from build123d import *

# Parameters (mm, degrees)
SKETCH2_W                   = 100
SKETCH2_H                   = 47
BOSS_EXTRUDE1_DEPTH         = 40
FILLET1_R                   = 10
CUT_EXTRUDE1_REACH          = 70.207
M6_TAPPED_HOLE1_D           = 5
M6_TAPPED_HOLE1_DEPTH       = 17
M6_TAPPED_HOLE1_CSINK_D     = 6.05
M6_TAPPED_HOLE1_CSINK_ANGLE = 90
M6_TAPPED_HOLE1_TIP         = 1.502151548


with BuildPart() as part:
    # Sketch2 → Boss-Extrude1 (new body)
    with BuildSketch(Plane(origin=(0, 0, 0), x_dir=(1, 0, 0), z_dir=(0, 1, 0))):
        Rectangle(SKETCH2_W, SKETCH2_H)
    extrude(amount=-BOSS_EXTRUDE1_DEPTH)

    # Fillet1
    fillet1_edges = [part.edges().sort_by_distance(p)[0] for p in [
        (50, -20, 23.5),
        (-50, -20, 23.5),
        (-50, -20, -23.5),
        (50, -20, -23.5),
    ]]
    fillet(fillet1_edges, radius=FILLET1_R)

    # Sketch3 → Cut-Extrude1 (cut, up to next)
    with BuildSketch(Plane(origin=(0, 0, 0), x_dir=(1, 0, 0), z_dir=(0, 1, 0)), mode=Mode.PRIVATE) as cut_extrude1_sk1:
        with BuildLine():
            Line((24.05, -10.14), (24.05, 10.14))
            ThreePointArc((24.05, 10.14), (23.156675683, 12.296675683), (21, 13.19))
            Line((21, 13.19), (-21, 13.19))
            ThreePointArc((-21, 13.19), (-23.156675683, 12.296675683), (-24.05, 10.14))
            Line((-24.05, 10.14), (-24.05, -10.14))
            ThreePointArc((-24.05, -10.14), (-23.156675683, -12.296675683), (-21, -13.19))
            Line((-21, -13.19), (-18.95, -13.19))
            Line((-18.95, -13.19), (-18.95, 8.09))
            Line((-18.95, 8.09), (18.95, 8.09))
            Line((18.95, 8.09), (18.95, -13.19))
            Line((18.95, -13.19), (21, -13.19))
            ThreePointArc((21, -13.19), (23.156675683, -12.296675683), (24.05, -10.14))
        make_face()
    cut_extrude1_tool1 = extrude(cut_extrude1_sk1.sketch, amount=-CUT_EXTRUDE1_REACH, mode=Mode.PRIVATE) & part.part
    add(cut_extrude1_tool1.solids().sort_by_distance((23.50141, 0, 0))[0], mode=Mode.SUBTRACT)

    # M6 Tapped Hole1
    with Locations(Plane(origin=(0, -40, 0), x_dir=(-1, 0, 0), z_dir=(0, -1, 0))):
        with Locations((-43, 16.5), (43, 16.5), (43, -16.5), (-43, -16.5)):
            CounterSinkHole(M6_TAPPED_HOLE1_D / 2, M6_TAPPED_HOLE1_CSINK_D / 2, depth=M6_TAPPED_HOLE1_DEPTH, counter_sink_angle=M6_TAPPED_HOLE1_CSINK_ANGLE)
            with Locations((0, 0, -(M6_TAPPED_HOLE1_DEPTH + M6_TAPPED_HOLE1_TIP / 2))):  # 118° drill point
                Cone(0, M6_TAPPED_HOLE1_D / 2, M6_TAPPED_HOLE1_TIP, mode=Mode.SUBTRACT)

    # Cut-Sweep1: sweep along a path in Sketch8
    with BuildLine(Plane(origin=(0, 0, 0), x_dir=(1, 0, 0), z_dir=(0, 1, 0))) as cut_sweep1_path:
        Line((18.95, 8.09), (18.95, -13.19))
        Line((18.95, -13.19), (21, -13.19))
        ThreePointArc((21, -13.19), (23.156675683, -12.296675683), (24.05, -10.14))
        Line((24.05, -10.14), (24.05, 10.14))
        ThreePointArc((24.05, 10.14), (23.156675683, 12.296675683), (21, 13.19))
        Line((21, 13.19), (-21, 13.19))
        ThreePointArc((-21, 13.19), (-23.156675683, 12.296675683), (-24.05, 10.14))
        Line((-24.05, 10.14), (-24.05, -10.14))
        ThreePointArc((-24.05, -10.14), (-23.156675683, -12.296675683), (-21, -13.19))
        Line((-21, -13.19), (-18.95, -13.19))
        Line((-18.95, -13.19), (-18.95, 8.09))
        Line((-18.95, 8.09), (18.95, 8.09))
    # Sketch7 → Cut-Sweep1 (sweep, cut)
    with BuildSketch(Plane(origin=(0, 0, 0), x_dir=(0, 0, -1), z_dir=(1, 0, 0))):
        Polygon((13.19, -3.2), (13.832346389, -40), (13.19, -40), align=None)
    sweep(path=cut_sweep1_path.line, transition=Transition.RIGHT, mode=Mode.SUBTRACT)


solid = part.part
Verification items for the finished model (mm, model axes). A direction names the side the tool comes from. Coordinates: 2 decimals unless noted, no trailing zeros. Loops run counter-clockwise (first coordinate to the right, second up) from the corner with the lowest first, then second, coordinate; pieces in that order, holes last. Notation, with made-up numbers: M 81.25,-32.75 L 96.25,-32.75 A24 cw 96.25,3.25 Z; hole C -30.75,-19.75 d6. An arc over 180 degrees is marked long. One line per item, written item: value.
1. Section check B-B on x = -3. Record the cut outline in (y, z).
Answers follow:
outline: M -40,-23.5 L 0,-23.5 L 0,-13.19 L -3.2,-13.19 L -40,-13.83 Z; M -40,-7.45 L -3.2,-8.09 L 0,-8.09 L 0,23.5 L -40,23.5 Z
2. Section check A-A on z = -3. Record the cut outline in (x, y).
Answers follow:
outline: M -50,-40 L -24.69,-40 L -24.05,-3.2 L -24.05,0 L -50,0 Z; M -18.95,-3.2 L -18.31,-40 L 18.31,-40 L 18.95,-3.2 L 18.95,0 L -18.95,0 Z; M 24.05,-3.2 L 24.69,-40 L 50,-40 L 50,0 L 24.05,0 Z
3. Section check C-C on y = -28. Record the cut outline in (x, z).
Answers follow:
outline: M -50,-13.5 A10 ccw -40,-23.5 L 40,-23.5 A10 ccw 50,-13.5 L 50,13.5 A10 ccw 40,23.5 L -40,23.5 A10 ccw -50,13.5 Z; hole C -43,-16.5 d5; hole C -43,16.5 d5; hole M -24.48,-10.14 A3.48 ccw -21,-13.62 L 21,-13.62 A3.48 ccw 24.48,-10.14 L 24.48,10.14 A3.48 ccw 21,13.62 L 18.52,13.62 L 18.52,-7.66 L -18.52,-7.66 L -18.52,13.62 L -21,13.62 A3.48 ccw -24.48,10.14 Z; hole C 43,-16.5 d5; hole C 43,16.5 d5
4. Material ranges on line 1 along Z through (x, y) = (-20.5, -2); line 2 along X through (y, z) = (-25.5, 4); line 3 along X through (y, z) = (-25, 17.5), recorded low to high. Write a range as from..to.
Answers follow:
line 1: -23.5..-13.19, 13.19..23.5
line 2: -50..-24.44, -18.56..18.56, 24.44..50
line 3: -49.17..-45.29, -40.71..40.71, 45.29..49.17
5. Section check D-D on y = -12. Record the cut outline in (x, z).
Answers follow:
outline: M -50,-13.5 A10 ccw -40,-23.5 L 40,-23.5 A10 ccw 50,-13.5 L 50,13.5 A10 ccw 40,23.5 L -40,23.5 A10 ccw -50,13.5 Z; hole M -24.2,-10.14 A3.2 ccw -21,-13.34 L 21,-13.34 A3.2 ccw 24.2,-10.14 L 24.2,10.14 A3.2 ccw 21,13.34 L 18.8,13.34 L 18.8,-7.94 L -18.8,-7.94 L -18.8,13.34 L -21,13.34 A3.2 ccw -24.2,10.14 Z
6. Mould release check, pull along X, two halves, no side actions. Record for faces 1 (the flat face through (-24.05, -2, 0)), 2 (the cylindrical face through (-47.15, -20.28, 20.49)), 3 (the flat face through (-1, -20, -23.5)): pulls with the +X half, pulls with the -X half, needs draft (parallel to the pull), parting line crosses it, or undercut.
Answers follow:
face 1: undercut
face 2: pulls with the -X half
face 3: needs draft
7. Set-up check for faces 4 (the conical face through (-23.4, -21.3, 12.5)), 5 (the flat face through (0, -2, -13.19)), 6 (the flat face through (-50, -20, 0)): record each of +Z, -Z, +X, -X, +Y, -Y from which the full face is reachable in a straight line by a thin tool's end or side.
Answers follow:
face 4: -Y
face 5: +Y, -Y
face 6: +Z, -Z, -X, +Y, -Y
8. Gauge pin test, flat end, axial feed: P1, Ø6, axis at x = -43, z = -16.5, coming from the -Y side (3 decimals). Record the tip position at first contact, or that the pin passes through.
Answers follow:
P1: y = -39.975
